Source: CAD feature listing. Evaluate the final solid. Frame: model axes, mm. A direction names the side the tool comes from. Coordinates: 2 decimals unless noted, no trailing zeros. Loops run counter-clockwise (first coordinate to the right, second up) from the corner with the lowest first, then second, coordinate; pieces in that order, holes last. Notation, with made-up numbers: M -27,32.5 L -7,32.5 A22 ccw -7,38.5 Z; hole C 41,-3 d5. An arc over 180 degrees is marked long. One line per question, with ' | ' between items. Start each with the question number.
1. Pin query (flat end, axial travel): P1, Ø1.5, axis at x = -5.5, y = -7.5, coming from the +Z side; P2, Ø3, axis at x = 9, y = -1, coming from the +Z side; P3, Ø3, axis at y = -3.5, z = 7.5, coming from the +X side. Return the tip coordinate at first contact, or that it passes through.
2. Section query A-A, the plane x = 0. Output: boundary loops of the cut face in (y, z), and give its area (4 significant figures).
3. Section query D-D, the plane x = -13.5. Output: boundary loops of the cut face in (y, z), and give its area (4 significant figures).
4. Section query C-C, the plane z = 0. Output: boundary loops of the cut face in (x, y).
5. Ray query, probe 1 along Z at (x, y) = (0, -1.5); probe 2 along X at (y, z) = (-3.5, 10). Return the intervals inside material, ascending.
6. Mould query, pull axis X, two halves, no side actions, for faces 1 (the flat face through (9.51, -7.23, -9.74)), 2 (the flat face through (-9.74, -7.23, -9.51)), 3 (the cylindrical face through (0, -4, -1)). Classes: pulls with the +X half, pulls with the -X half, needs draft (parallel to the pull), parting line crosses it, or undercut.
7. Access query for faces 4 (the flat face through (10, -3, -1.75)), 5 (the cylindrical face through (0, -8, -2)), 6 (the flat face through (-1.75, -3, 10)), 7 (the flat face through (1.75, -3, 10)), 8 (the flat face through (-1.75, -3, -10)). Directions: +Z, -Z, +X, -X, +Y, -Y. A direction counts if a zero-diameter tool reaches every point of the face in a straight line with its end or side. Return the directions, or none.
8. Section query B-B, the plane y = -3. Output: boundary loops of the cut face in (x, z), and give its area (3 significant figures).
```python
from build123d import *

# Parameters (mm, degrees)
F1_DEPTH = 6
F3_DEPTH = 2.5
F4_R     = 1
F5_DEPTH = 8.501
F6_R     = 2
F7_DEPTH = 1


with BuildPart() as f1:
    # F0 (on Front) → F1 (new body)
    with BuildSketch(Plane.XZ):
        Polygon((1.75, 1.75), (1.75, 17.5), (-1.75, 17.5), (-1.75, 1.75), (-17.5, 1.75), (-17.5, -1.75), (-1.75, -1.75), (-1.75, -17.5), (1.75, -17.5), (1.75, -1.75), (17.5, -1.75), (17.5, 1.75), align=None)
    extrude(amount=F1_DEPTH)

    # F2 (on face) → F3 (join)
    with BuildSketch(Plane.XZ.offset(6)):
        Polygon((-1.75, 17.5), (-17.5, 1.75), (-17.5, 0), (-17.5, -1.75), (-1.75, -17.5), (0, -17.5), (1.75, -17.5), (17.5, -1.75), (17.5, 0), (17.5, 1.75), (1.75, 17.5), (0, 17.5), align=None)
    extrude(amount=F3_DEPTH)

    # F4 (on face) → F5 (cut, through all)
    with BuildSketch(Plane(origin=(0, 0, 0), x_dir=(-1, 0, 0), z_dir=(0, 1, 0))):
        Circle(F4_R)
    extrude(amount=-F5_DEPTH, mode=Mode.SUBTRACT)

    # F6 (on face) → F7 (cut)
    with BuildSketch(Plane.XZ.offset(8.5)):
        Circle(F6_R)
    extrude(amount=-F7_DEPTH, mode=Mode.SUBTRACT)


solid = f1.part
```
Taken from the geometry:
1) P1: z = 14.5 | P2: z = 1.75 | P3: x = 1.75
2) outline: M -8.5,-17.5 L 0,-17.5 L 0,-1 L -7.5,-1 L -7.5,-2 L -8.5,-2 Z; M -8.5,2 L -7.5,2 L -7.5,1 L 0,1 L 0,17.5 L -8.5,17.5 Z | area: 278.5 mm^2
3) outline: M -8.5,-5.75 L -6,-5.75 L -6,-1.75 L 0,-1.75 L 0,1.75 L -6,1.75 L -6,5.75 L -8.5,5.75 Z | area: 49.75 mm^2
4) outline: M -17.5,-8.5 L -2,-8.5 L -2,-7.5 L -1,-7.5 L -1,0 L -17.5,0 Z; M 1,-7.5 L 2,-7.5 L 2,-8.5 L 17.5,-8.5 L 17.5,0 L 1,0 Z
5) probe 1: -17.5 to -1, 1 to 17.5 | probe 2: -1.75 to 1.75
6) face 1: pulls with the +X half | face 2: pulls with the -X half | face 3: undercut
7) face 4: -Z, +X, +Y | face 5: -Y | face 6: +Z, -X, +Y | face 7: +Z, +X, +Y | face 8: -Z, -X, +Y
8) outline: M -17.5,-1.75 L -1.75,-1.75 L -1.75,-17.5 L 1.75,-17.5 L 1.75,-1.75 L 17.5,-1.75 L 17.5,1.75 L 1.75,1.75 L 1.75,17.5 L -1.75,17.5 L -1.75,1.75 L -17.5,1.75 Z; hole C 0,0 d2 | area: 230 mm^2
